Part model, mm, in its own coordinate system. Face numbers are marked on the shaded views. Round coordinates to 2 decimals unless told otherwise and drop trailing zeros. Write each loop counter-clockwise with the first axis right and the second up, starting at its lowest first coordinate (ties: lowest second). Pieces come first, ordered by that corner, then holes. Notation, with made-up numbers: (-5.75, 70.25) -> (-0.75, 70.25) arc R29 ccw to (-0.75, 100.25) -> close; hole circle Ø1 at (-7.75, 64.5). An arc over 180 degrees is marked (long way). Use CSV: the item, a comma, the result in double quotes. Start each with the question number.
(1) Saw through at A-A (x = 127). Give the cut face in (y, z), plus the area to 3 significant figures.
(2) Saw through at C-C (y = 29.5). Give the cut face in (x, z).
(3) Two-plate mould, pull along X, no slides. Class the marked faces 1, 2, 3 and 4: released by +X, released by -X, zero draft, split by the parting line, or undercut.
(4) Drop flat-ended pins along their axis: pin 1 (4 mm diameter, centred on x = 209, z = 2.5, fed in from +Y); pin 2 (4 mm diameter, centred on x = 163.5, y = 30.5, fed in from +Z); pin 3 (4 mm diameter, centred on x = 222.5, z = 3, fed in from +Y); pin 4 (1.5 mm diameter, centred on x = 158.5, z = 8, fed in from -Y). Give the stop position or say it passes through.
(5) Probe line 1 (X direction, y = 22, z = 11.5); line 2 (X direction, y = 12, z = 2.75); line 3 (Y direction, x = 241.3, z = 6). List the from-to ranges inside material, lowest first. Write a range as [from, to].
(6) Saw through at B-B (z = 7.25). Give the cut face in (x, y).
(7) Saw through at D-D (y = 12.7). Give the cut face in (x, z).
```python
from build123d import *

# Parameters (mm, degrees)
F0_R     = 2.15265
F1_DEPTH = 12.7


with BuildPart() as f1:
    # F0 (on Top) → F1 (new body)
    with BuildSketch(Plane.XY):
        with BuildLine():
            ThreePointArc((248.92, 22.86), (127, 63.5), (5.08, 22.86))
            ThreePointArc((5.08, 22.86), (2.54, 5.08), (20.32, 2.54))
            ThreePointArc((20.32, 2.54), (127, 38.1), (233.68, 2.54))
            ThreePointArc((233.68, 2.54), (251.46, 5.08), (248.92, 22.86))
        make_face()
        with Locations((12.7, 12.7)):
            Circle(F0_R, mode=Mode.SUBTRACT)
        with Locations((241.3, 12.7)):
            Circle(F0_R, mode=Mode.SUBTRACT)
        with Locations((127, 50.8)):
            Circle(F0_R, mode=Mode.SUBTRACT)
    extrude(amount=F1_DEPTH)


solid = f1.part
```
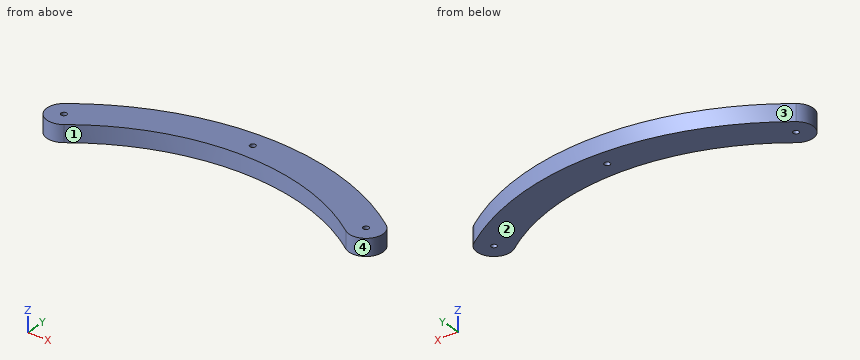
Answers:
1,outline,"(38.1, 0) -> (48.65, 0) -> (48.65, 12.7) -> (38.1, 12.7) -> close; (52.95, 0) -> (63.5, 0) -> (63.5, 12.7) -> (52.95, 12.7) -> close"
1,area,"268 mm²"
2,outline,"(14.48, 0) -> (72.37, 0) -> (72.37, 12.7) -> (14.48, 12.7) -> close; (181.63, 0) -> (239.52, 0) -> (239.52, 12.7) -> (181.63, 12.7) -> close"
3,face 1,"undercut"
3,face 2,"zero draft"
3,face 3,"split by the parting line"
3,face 4,"undercut"
4,pin 1,"stops at y = 47.09"
4,pin 2,"passes through"
4,pin 3,"stops at y = 40.71"
4,pin 4,"stops at y = 35.15"
5,line 1,"x = [4.05, 53.07], [200.93, 249.95]"
5,line 2,"x = [0.02, 10.66], [14.74, 34.26], [219.74, 239.26], [243.34, 253.98]"
5,line 3,"y = [0, 10.55], [14.85, 28.31]"
6,outline,"(5.08, 22.86) arc R12.7 ccw to (20.32, 2.54) arc R177.8 cw to (233.68, 2.54) arc R12.7 ccw to (248.92, 22.86) arc R203.2 ccw to start; hole circle Ø4.31 at (12.7, 12.7); hole circle Ø4.31 at (127, 50.8); hole circle Ø4.31 at (241.3, 12.7)"
7,outline,"(0, 0) -> (10.55, 0) -> (10.55, 12.7) -> (0, 12.7) -> close; (14.85, 0) -> (35.42, 0) -> (35.42, 12.7) -> (14.85, 12.7) -> close; (218.58, 0) -> (239.15, 0) -> (239.15, 12.7) -> (218.58, 12.7) -> close; (243.45, 0) -> (254, 0) -> (254, 12.7) -> (243.45, 12.7) -> close"
